from build123d import *

# Parameters (mm, degrees)
F0_W     = 16
F0_H     = 130
F1_DEPTH = 10
F2_R     = 5
F3_DEPTH = 11
F4_W     = 10
F4_H     = 16
F5_DEPTH = 5
F6_R     = 7.99999
F7_R     = 4.99999
F8_R     = 2.5


# Not quite as in the source:
# - a fillet or chamfer is up to 0.001 mm smaller than in the source, because OpenCascade refuses the exact size


with BuildPart() as f1:
    # F0 (on Right) → F1 (new body)
    with BuildSketch(Plane.YZ):
        with Locations((0, -57)):
            Rectangle(F0_W, F0_H)
    extrude(amount=F1_DEPTH)

    # F2 (on face) → F3 (join)
    with BuildSketch(Plane.YZ.offset(10)):
        Circle(F2_R)
    extrude(amount=F3_DEPTH)

    # F4 (on face) → F5 (join)
    with BuildSketch(Plane.YZ.offset(21)):
        Rectangle(F4_W, F4_H)
    extrude(amount=F5_DEPTH)

    # F6 (radius 8 in the source; OpenCascade refuses exactly that, so slightly less here)
    f6_edges = [f1.edges().sort_by_distance(p)[0] for p in [
        (5, -8, 8),
        (5, 8, 8),
    ]]
    fillet(f6_edges, radius=F6_R)

    # F7 (radius 5 in the source; OpenCascade refuses exactly that, so slightly less here)
    f7_edges = [f1.edges().sort_by_distance(p)[0] for p in [
        (23.5, -5, 8),
        (23.5, 5, 8),
        (23.5, -5, -8),
        (23.5, 5, -8),
    ]]
    fillet(f7_edges, radius=F7_R)

    # F8
    f8_edges = [f1.edges().sort_by_distance(p)[0] for p in [
        (26, 3.535537, 6.535537),
        (10, -5.656857, 5.656857),
        (0, -5.656857, 5.656857),
        (0, 0, -122),
        (5, -8, -122),
        (10, 0, -122),
        (5, 8, -122),
    ]]
    fillet(f8_edges, radius=F8_R)


solid = f1.part
Verification items for the finished model (mm, model axes). A direction names the side the tool comes from. Coordinates: 2 decimals unless noted, no trailing zeros. Loops run counter-clockwise (first coordinate to the right, second up) from the corner with the lowest first, then second, coordinate; pieces in that order, holes last. Notation, with made-up numbers: M 38.25,-2.75 L 43.25,-2.75 A18 ccw 43.25,11.25 Z; hole C 58.25,26 d3. An arc over 180 degrees is marked long. One line per item, written item: value.
1. Gauge pin test, flat ends, axial feed: P1, Ø2, axis at x = 16.5, y = -4, coming from the -Z side; P2, Ø3, axis at x = 22, z = -1.5, coming from the -Y side; P3, Ø1.2, axis at x = 22.5, z = 0.5, coming from the +Y side. Record the tip position at first contact, or that the pin passes through.
Answers follow:
P1: z = -4
P2: y = -5
P3: y = 5
2. Material ranges on line 1 along X through (y, z) = (-5.75, -32); line 2 along Z through (x, y) = (19.75, -4); line 3 along Z through (x, y) = (19, 0), recorded low to high. Write a range as from..to.
Answers follow:
line 1: 0.01..9.99
line 2: -3..3
line 3: -5..5
3. Section check B-B on x = 19.25. Record the cut outline in (y, z).
Answers follow:
outline: C 0,0 d10
4. Mould release check, pull along Z, two halves, no side actions. Record for faces 1 (the cylindrical face through (15.42, -1.08, -4.88)), 2 (the flat face through (21, 0, 6)), 3 (the cylindrical face through (0.752, 0.077, -121.287)), 4 (the cylindrical face through (5.035, 5.594, 5.719)): pulls with the +Z half, pulls with the -Z half, needs draft (parallel to the pull), parting line crosses it, or undercut.
Answers follow:
face 1: parting line crosses it
face 2: needs draft
face 3: pulls with the -Z half
face 4: pulls with the +Z half
5. Section check A-A on z = -44.5. Record the cut outline in (x, y).
Answers follow:
outline: M 0,-5.5 A2.5 ccw 2.5,-8 L 7.5,-8 A2.5 ccw 10,-5.5 L 10,5.5 A2.5 ccw 7.5,8 L 2.5,8 A2.5 ccw 0,5.5 Z
6. Set-up check for faces 5 (the flat face through (21, 0, -6)), 6 (the flat face through (22, -5, 0)), 7 (the cylindrical face through (22, 4, -6)), 8 (the flat face through (22, 5, 0)): record each of +Z, -Z, +X, -X, +Y, -Y from which the full face is reachable in a straight line by a thin tool's end or side.
Answers follow:
face 5: -Z, +Y
face 6: +Z, -Z, +X, -Y
face 7: -Z, +X, +Y
face 8: +Z, -Z, +X, +Y
